Check sheet for the modelled part. Datum: model origin and axes. Units: mm. Face numbers are marked on the shaded views. A direction names the side the tool comes from. Round coordinates to 2 decimals unless told otherwise and drop trailing zeros. Loops run counter-clockwise (first coordinate to the right, second up) from the corner with the lowest first, then second, coordinate; pieces in that order, holes last. Notation, with made-up numbers: (38.5, 48.25) -> (57.5, 48.25) arc R27 cw to (57.5, 69.25) -> close; hole circle Ø10 at (65.25, -34.75). An arc over 180 degrees is marked (long way). One line per question, with ' | ' between items.
```python
from build123d import *

# Parameters (mm, degrees)
ESQUISSE1_R             = 3
BASE_EXTRUSION_DEPTH    = 15
ESQUISSE2_R             = 5
BOSS_EXTRU_1_DEPTH      = 6
ENL_V_MAT_EXTRU_1_DEPTH = 4
CHANFREIN3_SIZE         = 0.2
CONG_1_R                = 0.3


with BuildPart() as part:
    # Esquisse1 → Base-Extrusion (new body)
    with BuildSketch(Plane.XY):
        Circle(ESQUISSE1_R)
    extrude(amount=BASE_EXTRUSION_DEPTH)

    # Esquisse2 → Boss.-Extru.1 (add)
    with BuildSketch(Plane.XY.offset(15)):
        Circle(ESQUISSE2_R)
    extrude(amount=BOSS_EXTRU_1_DEPTH)

    # Esquisse3 → Enlèv. mat.-Extru.1 (cut)
    with BuildSketch(Plane.XY.offset(21)):
        Polygon((-3, 0), (-1.500108314, 2.598013673), (1.500108314, 2.598013673), (3, 0), (1.500108314, -2.598013673), (-1.500108314, -2.598013673), align=None)
    extrude(amount=-ENL_V_MAT_EXTRU_1_DEPTH, mode=Mode.SUBTRACT)

    # Chanfrein3
    chanfrein3_edges = [part.edges().sort_by_distance(p)[0] for p in [
        (-2.250054157, -1.299006837, 21),
        (0, -2.598013673, 21),
        (2.250054157, -1.299006837, 21),
        (2.250054157, 1.299006837, 21),
        (0, 2.598013673, 21),
        (-2.250054157, 1.299006837, 21),
    ]]
    chamfer(chanfrein3_edges, length=CHANFREIN3_SIZE)

    # Congé1
    cong_1_edges = [part.edges().sort_by_distance(p)[0] for p in [
        (-5, 0, 21),
    ]]
    fillet(cong_1_edges, radius=CONG_1_R)


solid = part.part
```
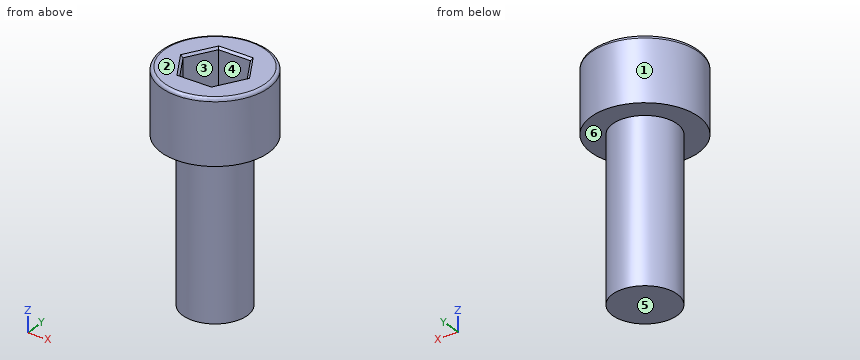
(1) Set-up check for the marked faces 4, 5 and 6: record each of +Z, -Z, +X, -X, +Y, -Y from which the full face is reachable in a straight line by a thin tool's end or side.
Answer:
face 4: +Z | face 5: -Z, +X, -X, +Y, -Y | face 6: -Z
(2) Mould release check, pull along X, two halves, no side actions. Record for the marked faces 1, 2 and 3: +X half, -X half, draft (parallel to the pull), parting line (faces both ways), or undercut.
Answer:
face 1: parting line | face 2: draft | face 3: undercut
(3) Sectioned sample at B-B, the plane z = 13. Record the cut outline in (x, y), and give its area (3 significant figures).
Answer:
outline: circle Ø6 at (0, 0) | area: 28.3 mm2
(4) Scan lines: probe 1 along Z at (x, y) = (1.75, 2); probe 2 along Y at (x, z) = (-1.5, 11.25); probe 3 along Z at (x, y) = (1.75, -3.25). Record each from-to range of solid material in increasing order.
Answer:
probe 1: z = 0 to 17 | probe 2: y = -2.6 to 2.6 | probe 3: z = 15 to 21
(5) Sectioned sample at A-A, the plane x = 0. Record the cut outline in (y, z).
Answer:
outline: (-5, 15) -> (-3, 15) -> (-3, 0) -> (3, 0) -> (3, 15) -> (5, 15) -> (5, 20.7) arc R0.3 ccw to (4.7, 21) -> (2.8, 21) -> (2.6, 20.8) -> (2.6, 17) -> (-2.6, 17) -> (-2.6, 20.8) -> (-2.8, 21) -> (-4.7, 21) arc R0.3 ccw to (-5, 20.7) -> close
